Work out the finished part from the listing and answer in its coordinate system (mm). Face numbers are marked on the shaded views. A direction names the side the tool comes from. Coordinates: 2 decimals unless noted, no trailing zeros. Write each loop counter-clockwise with the first axis right and the second up, starting at its lowest first coordinate (ties: lowest second). Pieces come first, ordered by that corner, then holes. Notation, with made-up numbers: M -38,52.25 L 10,52.25 A26 ccw 10,80.25 Z; hole C -7.5,81.5 d4. An arc over 180 degrees is marked long. Use CSV: the item, a comma, the result in double quotes.
from build123d import *

# Parameters (mm, degrees)
SKETCH1_R                      = 15
EXTRUDE1_DEPTH                 = 17
EXTRUDE3_DEPTH                 = 17
CIRPATTERN1_COUNT              = 20
F_8_2_8_2_DIAMETER_HOLE1_D     = 8.2
F_8_2_8_2_DIAMETER_HOLE1_DEPTH = 10
F_8_2_8_2_DIAMETER_HOLE1_TIP   = 2.463528538
EXTRUDE5_DEPTH                 = 14
SKETCH7_R                      = 1.95
EXTRUDE6_DEPTH                 = 15


with BuildPart() as part:
    # Sketch1 → Extrude1 (new body)
    with BuildSketch(Plane.XY):
        Circle(SKETCH1_R)
    extrude(amount=EXTRUDE1_DEPTH)

    # Sketch2 → Extrude3 (add)
    with BuildSketch(Plane.XY.offset(17)):
        Polygon((1.4, 14.704480908), (1, 16.404480908), (-1, 16.404480908), (-1.4, 14.704480908), align=None)
    extrude3 = extrude(amount=-EXTRUDE3_DEPTH)

    # CirPattern1: Extrude3 ×20 about axis
    cirpattern1_axis = Axis((0, 0, 0), (0, 0, 1))
    for i in range(1, CIRPATTERN1_COUNT):
        add(extrude3.rotate(cirpattern1_axis, i * 360 / CIRPATTERN1_COUNT))

    # Ø8.2 (8.2) Diameter Hole1
    with Locations(Plane(origin=(0, 0, 0), x_dir=(-1, 0, 0), z_dir=(0, 0, -1))):
        with Locations((0, 0)):
            Hole(F_8_2_8_2_DIAMETER_HOLE1_D / 2, depth=F_8_2_8_2_DIAMETER_HOLE1_DEPTH)
            with Locations((0, 0, -(F_8_2_8_2_DIAMETER_HOLE1_DEPTH + F_8_2_8_2_DIAMETER_HOLE1_TIP / 2))):  # 118° drill point
                Cone(0, F_8_2_8_2_DIAMETER_HOLE1_D / 2, F_8_2_8_2_DIAMETER_HOLE1_TIP, mode=Mode.SUBTRACT)

    # Sketch6 → Extrude5 (cut)
    with BuildSketch(Plane.XY.offset(17)):
        Polygon((4.053764157, 6.992877054), (-4.029127096, 7.007101268), (-8.082891253, 0.014224214), (-4.053764157, -6.992877054), (4.029127096, -7.007101268), (8.082891253, -0.014224214), align=None)
    extrude(amount=-EXTRUDE5_DEPTH, mode=Mode.SUBTRACT)

    # Sketch7 → Extrude6 (cut)
    with BuildSketch(Plane.XY.offset(17)):
        with Locations((-11, 0)):
            Circle(SKETCH7_R)
        with Locations((0, 11)):
            Circle(SKETCH7_R)
        with Locations((11, 0)):
            Circle(SKETCH7_R)
        with Locations((0, -11)):
            Circle(SKETCH7_R)
    extrude(amount=-EXTRUDE6_DEPTH, mode=Mode.SUBTRACT)


solid = part.part
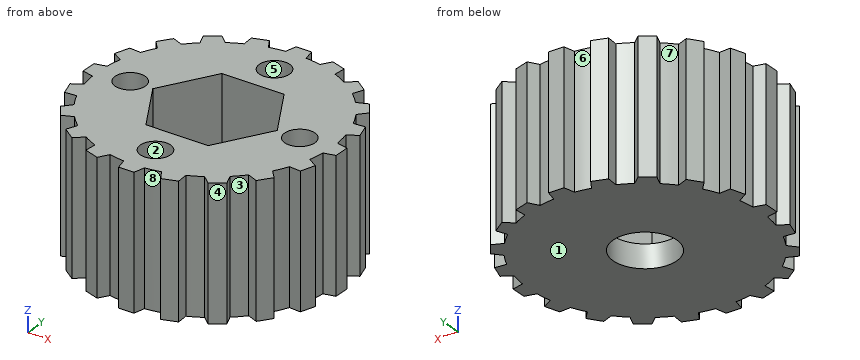
Item 1: The part is cut by section A-A (x = 0). Write down the section's boundary in (y, z).
Answer:
outline,"M -16.4,0 L -4.1,0 L -4.1,3 L -7,3 L -7,17 L -9.05,17 L -9.05,2 L -12.95,2 L -12.95,17 L -16.4,17 Z; M 4.1,0 L 16.4,0 L 16.4,17 L 12.95,17 L 12.95,2 L 9.05,2 L 9.05,17 L 7,17 L 7,3 L 4.1,3 Z"
Item 2: Consider probe 1 along Y at (x, z) = (0, 12); probe 2 along Y at (x, z) = (13.5, 9.75); probe 3 along X at (y, z) = (0.5, 5.5). Determine where each line is inside the solid, lowest interval first.
Answer:
probe 1,"y = -16.4 to -12.95, -9.05 to -7, 7 to 9.05, 12.95 to 16.4"
probe 2,"y = -9.33 to -8.42, -6.54 to 6.54, 8.42 to 9.33"
probe 3,"x = -16.4 to -12.88, -9.12 to -7.8, 7.79 to 9.12, 12.88 to 16.4"
Item 3: Given pin 1 (3 mm diameter, centred on x = 11, y = 0, fed in from +Z); pin 2 (1 mm diameter, centred on y = -5, z = 3.5, fed in from -X); pin 3 (6 mm diameter, centred on x = 7, z = 5.5, fed in from +Y), each flat-ended and moving along its own axis, determine where each tip first touches the part or whether it passes through.
Answer:
pin 1,"stops at z = 2"
pin 2,"stops at x = -15.79"
pin 3,"stops at y = 15.91"
Item 4: The part is cut by section B-B (z = 15). Count the separate pieces of the cut face and the enclosed holes in it, then the cut area to 3 significant figures.
Answer:
separate pieces,"1"
enclosed holes,"5"
area,"556 mm2"
Item 5: For a pull along Y with two mould halves and no side action, classify the marked faces 1, 2, 3 and 4 as released by +Y, released by -Y, zero draft, split by the parting line, or undercut.
Answer:
face 1,"zero draft"
face 2,"undercut"
face 3,"undercut"
face 4,"released by -Y"
Item 6: The part is cut by section C-C (x = -7). Write down the section's boundary in (y, z).
Answer:
outline,"M -13.27,0 L 13.27,0 L 13.27,17 L 1.88,17 L 1.88,3 L -1.87,3 L -1.87,17 L -13.27,17 Z"
Item 7: A tool of negligible diameter and unlimited length cuts with its end or side. For the marked faces 5, 6, 7 and 8, from which of +Z, -Z, +X, -X, +Y, -Y can it reach the whole face along a straight path? Write none if from no direction.
Answer:
face 5,"+Z"
face 6,"+Z, -Z, +Y"
face 7,"+Z, -Z"
face 8,"+Z, -Z, -Y"
